The listing builds one solid part. Answer for the finished solid, in the listing's coordinates (mm). Face numbers are marked on the shaded views. Give positions to 0.01 mm unless a question says otherwise; leave off trailing zeros. Order: outer loops, then holes, each group sorted by start corner. A loop starts at its lowest first (then second) coordinate and runs counter-clockwise, first axis right, second up. Notation, with made-up numbers: (17.25, 30) -> (43.25, 30) arc R24 cw to (43.25, 41) -> close; hole circle Ø8 at (-22.5, 63.5). An arc over 180 degrees is marked (long way). One line per question, with ' | ' between items. Start each with the question number.
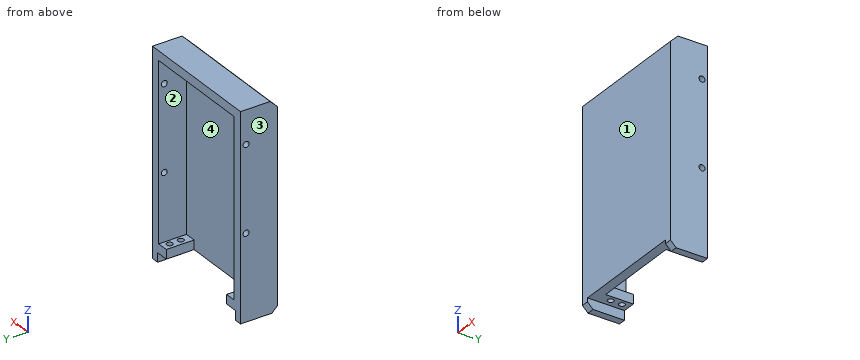
```python
from build123d import *

# Parameters (mm, degrees)
CROQUIS1_W                 = 70
CROQUIS1_H                 = 105
SALIENTE_EXTRUIR1_DEPTH    = 20
VACIADO1_T                 = -5
CROQUIS3_R                 = 1.6
CORTAR_EXTRUIR1_DEPTH      = 70
CROQUIS4_W                 = 60
CROQUIS4_H                 = 15
CORTAR_EXTRUIR2_DEPTH      = 5
CROQUIS5_W                 = 5
CROQUIS5_H                 = 15
SALIENTE_EXTRUIR2_DEPTH    = 6
CORTAR_EXTRUIR3_REACH      = 114.472
CROQUIS6_R                 = 1.6
CROQUIS7_W                 = 4
CROQUIS7_H                 = 5
SALIENTE_EXTRUIR3_DEPTH    = 20
CHAFL_N1_SIZE              = 3
CHAFL_N1_OF_SIMETR_A3_SIZE = 3
CHAFL_N2_SIZE              = 4


with BuildPart() as part:
    # Croquis1 → Saliente-Extruir1 (new body)
    with BuildSketch(Plane(origin=(0, 0, 0), x_dir=(1, 0, 0), z_dir=(0, 1, 0))):
        Rectangle(CROQUIS1_W, CROQUIS1_H)
    extrude(amount=SALIENTE_EXTRUIR1_DEPTH)

    # Vaciado1
    vaciado1_openings = [part.faces().sort_by_distance(p)[0] for p in [
        (0, 20, 0),
    ]]
    offset(amount=VACIADO1_T, openings=vaciado1_openings, kind=Kind.INTERSECTION)

    # Croquis3 → Cortar-Extruir1 (cut)
    with BuildSketch(Plane.ZY.offset(35)):
        with Locations((34.5, 17)):
            Circle(CROQUIS3_R)
        with Locations((-11.5, 17)):
            Circle(CROQUIS3_R)
    extrude(amount=-CORTAR_EXTRUIR1_DEPTH, mode=Mode.SUBTRACT)

    # Croquis4 → Cortar-Extruir2 (cut)
    with BuildSketch(Plane(origin=(0, 0, -52.5), x_dir=(-1, 0, 0), z_dir=(0, 0, -1))):
        with Locations((0, 12.5)):
            Rectangle(CROQUIS4_W, CROQUIS4_H)
    extrude(amount=-CORTAR_EXTRUIR2_DEPTH, mode=Mode.SUBTRACT)

    # Croquis5 → Saliente-Extruir2 (add)
    with BuildSketch(Plane(origin=(-30, 0, 0), x_dir=(0, 0, -1), z_dir=(1, 0, 0))):
        with Locations((50, 12.5)):
            Rectangle(CROQUIS5_W, CROQUIS5_H)
    saliente_extruir2 = extrude(amount=SALIENTE_EXTRUIR2_DEPTH)

    # Simetría1: Saliente-Extruir2 across plane
    add(saliente_extruir2.mirror(Plane(origin=(0, 0, 0), x_dir=(0, 0, 1), z_dir=(1, 0, 0))))

    # Croquis6 → Cortar-Extruir3 (cut, up to next)
    with BuildSketch(Plane(origin=(0, 0, -52.5), x_dir=(-1, 0, 0), z_dir=(0, 0, -1)), mode=Mode.PRIVATE) as cortar_extruir3_sk1:
        with Locations((-27.2, 16)):
            Circle(CROQUIS6_R)
    cortar_extruir3_tool1 = extrude(cortar_extruir3_sk1.sketch, amount=-CORTAR_EXTRUIR3_REACH, mode=Mode.PRIVATE) & part.part
    # Croquis6 → Cortar-Extruir3 (cut, up to next)
    with BuildSketch(Plane(origin=(0, 0, -52.5), x_dir=(-1, 0, 0), z_dir=(0, 0, -1)), mode=Mode.PRIVATE) as cortar_extruir3_sk2:
        with Locations((-27.2, 10)):
            Circle(CROQUIS6_R)
    cortar_extruir3_tool2 = extrude(cortar_extruir3_sk2.sketch, amount=-CORTAR_EXTRUIR3_REACH, mode=Mode.PRIVATE) & part.part
    cortar_extruir3_1 = cortar_extruir3_tool1.solids().sort_by_distance((27.2, 16, -52.5))[0]
    add(cortar_extruir3_1, mode=Mode.SUBTRACT)
    cortar_extruir3_2 = cortar_extruir3_tool2.solids().sort_by_distance((27.2, 10, -52.5))[0]
    add(cortar_extruir3_2, mode=Mode.SUBTRACT)
    cortar_extruir3 = cortar_extruir3_1 + cortar_extruir3_2  # Cortar-Extruir3 as one shape, for the pattern or mirror that repeats it

    # Simetría2: Cortar-Extruir3 across plane
    add(cortar_extruir3.mirror(Plane(origin=(0, 0, 0), x_dir=(0, 0, 1), z_dir=(1, 0, 0))), mode=Mode.SUBTRACT)

    # Croquis7 → Saliente-Extruir3 (add)
    with BuildSketch(Plane(origin=(0, 0, 0), x_dir=(1, 0, 0), z_dir=(0, 1, 0))):
        with Locations((33, 55)):
            Rectangle(CROQUIS7_W, CROQUIS7_H)
    saliente_extruir3 = extrude(amount=SALIENTE_EXTRUIR3_DEPTH)

    # Chaflán1
    chafl_n1_edges = [part.edges().sort_by_distance(p)[0] for p in [
        (33, 0, -57.5),
    ]]
    chamfer(chafl_n1_edges, length=CHAFL_N1_SIZE)

    # Simetría3: Saliente-Extruir3 across plane
    add(saliente_extruir3.mirror(Plane(origin=(0, 0, 0), x_dir=(0, 0, 1), z_dir=(1, 0, 0))))

    # Chaflán1 of Simetría3
    chafl_n1_of_simetr_a3_edges = [part.edges().sort_by_distance(p)[0] for p in [
        (-33, 0, -57.5),
    ]]
    chamfer(chafl_n1_of_simetr_a3_edges, length=CHAFL_N1_OF_SIMETR_A3_SIZE)

    # Chaflán2
    chafl_n2_edges = [part.edges().sort_by_distance(p)[0] for p in [
        (0, 0, 52.5),
    ]]
    chamfer(chafl_n2_edges, length=CHAFL_N2_SIZE)


solid = part.part
```
(1) The part is cut by section C-C on z = 4. Determine the outline of the cut face in (x, y).
(2) Determine the mould class of the marked faces 1, 2, 3 and 4 for opening direction X: pulls with the +X half, pulls with the -X half, needs draft (parallel to the pull), parting line crosses it, or undercut.
(3) The part is cut by section A-A on x = -27.2. Determine the outline of the cut face in (y, z), plus the area to 3 significant figures.
(4) Given P1, Ø2, axis at x = 7.5, z = -44.5, coming from the +Y side; P2, Ø1.9, axis at y = 17, z = 34.5, coming from the +X side; P3, Ø2.5, axis at x = 27.2, y = 16, coming from the -Z side; P4, Ø4, axis at x = 27.2, y = 10, coming from the -Z side, each flat-ended and moving along its own axis, determine where each tip first touches the part or whether it passes through.
(5) Consider line 1 (Y direction, x = -27.2, z = -49.1); line 2 (X direction, y = 12, z = 30.5); line 3 (Z direction, x = -7.5, y = 11.5). Determine where each line is inside the solid, lowest interval first.
(6) The part is cut by section B-B on z = -11.5. Determine the outline of the cut face in (x, y), plus the area to 3 significant figures.
(7) The part is cut by section D-D on x = 1.5. Determine the outline of the cut face in (y, z).
Result sheet:
1) outline: (-35, 0) -> (35, 0) -> (35, 20) -> (30, 20) -> (30, 5) -> (-30, 5) -> (-30, 20) -> (-35, 20) -> close
2) face 1: needs draft | face 2: undercut | face 3: pulls with the -X half | face 4: undercut
3) outline: (0, -52.5) -> (8.4, -52.5) -> (8.4, -47.5) -> (5, -47.5) -> (5, 47.5) -> (20, 47.5) -> (20, 52.5) -> (4, 52.5) -> (0, 48.5) -> close; (11.6, -52.5) -> (14.4, -52.5) -> (14.4, -47.5) -> (11.6, -47.5) -> close; (17.6, -52.5) -> (20, -52.5) -> (20, -47.5) -> (17.6, -47.5) -> close | area: 635 mm^2
4) P1: stops at y = 5 | P2: passes through | P3: stops at z = 47.5 | P4: stops at z = -52.5
5) line 1: y = 0 to 8.4, 11.6 to 14.4, 17.6 to 20 | line 2: x = -35 to -30, 30 to 35 | line 3: z = 47.5 to 52.5
6) outline: (-35, 0) -> (35, 0) -> (35, 15.4) -> (30, 15.4) -> (30, 5) -> (-30, 5) -> (-30, 15.4) -> (-35, 15.4) -> close; (-35, 18.6) -> (-30, 18.6) -> (-30, 20) -> (-35, 20) -> close; (30, 18.6) -> (35, 18.6) -> (35, 20) -> (30, 20) -> close | area: 468 mm^2
7) outline: (0, -52.5) -> (5, -52.5) -> (5, 47.5) -> (20, 47.5) -> (20, 52.5) -> (4, 52.5) -> (0, 48.5) -> close
